```python
from build123d import *

# Parameters (mm, degrees)
F0_W     = 6.3
F0_H     = 3.3
F1_DEPTH = 6.2
F3_R     = 3.15
F4_DEPTH = 3.5
F5_R     = 2.5
F6_DEPTH = 1
F7_R     = 3.15
F8_DEPTH = 6


with BuildPart() as f1:
    # F0 (on Top) → F1 (new body)
    with BuildSketch(Plane.XY):
        with Locations((0, -0.85)):
            Rectangle(F0_W, F0_H)
    extrude(amount=F1_DEPTH)

    # F3 (on offset) → F4 (join)
    with BuildSketch(Plane.XY.offset(3.8)):
        Circle(F3_R)
    extrude(amount=F4_DEPTH)

    # F5 (on face) → F6 (join)
    with BuildSketch(Plane.XY.offset(7.3)):
        Circle(F5_R)
    extrude(amount=F6_DEPTH)

    # F7 (on face) → F8 (join)
    with BuildSketch(Plane.XY.offset(8.3)):
        Circle(F7_R)
    extrude(amount=F8_DEPTH)


solid = f1.part
```
CAD build for the part. Positions are in the model's coordinates, mm. A direction names the side the tool comes from. Coordinates: 2 decimals unless noted, no trailing zeros. Order: outer loops, then holes, each group sorted by start corner. A loop starts at its lowest first (then second) coordinate and runs counter-clockwise, first axis right, second up. Notation, with made-up numbers: M 84.25,26 L 89.25,26 A29 cw 89.25,51 Z; hole C 13,-25.5 d6. An arc over 180 degrees is marked long. Answer as CSV lines item,"result".
1) Cut at D-D (z = 12). List the corners of the cut face in (x, y), then the cut area to 3 significant figures.
Verdict:
outline,"C 0,0 d6.3"
area,"31.2 mm2"
2) Cut at C-C (y = -1). List the corners of the cut face in (x, z).
Verdict:
outline,"M -3.15,0 L 3.15,0 L 3.15,6.2 L 2.99,6.2 L 2.99,7.3 L 2.29,7.3 L 2.29,8.3 L 2.99,8.3 L 2.99,14.3 L -2.99,14.3 L -2.99,8.3 L -2.29,8.3 L -2.29,7.3 L -2.99,7.3 L -2.99,6.2 L -3.15,6.2 Z"
3) 3-axis set-ups, long thin cutter, end or side, ignore diameter. For faces 1 (the flat face through (-2.8, -1.9, 6.2)), 2 (the flat face through (-2, 2, 7.3)), 3 (the flat face through (0, 2, 3.8)), 4 (the flat face through (2.8, -1.9, 6.2)): which of +Z, -Z, +X, -X, +Y, -Y reach the whole face in a straight line?
Verdict:
face 1,"+Z, -X, -Y"
face 2,"none"
face 3,"-Z, +X, -X, +Y"
face 4,"+Z, +X, -Y"
4) Drill centre lines: L1, parallel to Z at x = -2, y = -2; L2, parallel to Z at x = 1.75, y = 2.25; L3, parallel to Z at x = -1, y = 1. Where is each one in solid material? Low to high. Write a range as from..to.
Verdict:
L1,"0..7.3, 8.3..14.3"
L2,"3.8..7.3, 8.3..14.3"
L3,"3.8..14.3"
5) Flat gauge pins, fed straight in: P1, Ø0.5, axis at x = -0.5, y = -2.5, coming from the -Z side; P2, Ø1, axis at x = 2, z = 9.5, coming from the -Y side. Where does each tip first touch, or does it go through?
Verdict:
P1,"z = 0"
P2,"y = -2.77"
6) Cut at A-A (x = 0). List the corners of the cut face in (y, z), then the cut area to 3 significant figures.
Verdict:
outline,"M -3.15,3.8 L -2.5,3.8 L -2.5,0 L 0.8,0 L 0.8,3.8 L 3.15,3.8 L 3.15,7.3 L 2.5,7.3 L 2.5,8.3 L 3.15,8.3 L 3.15,14.3 L -3.15,14.3 L -3.15,8.3 L -2.5,8.3 L -2.5,7.3 L -3.15,7.3 Z"
area,"77.4 mm2"
7) Cut at B-B (z = 1.25). List the corners of the cut face in (x, y).
Verdict:
outline,"M -3.15,-2.5 L 3.15,-2.5 L 3.15,0.8 L -3.15,0.8 Z"
